```python
from build123d import *

# Parameters (mm, degrees)
BOSS_EXTRUDE1_DEPTH = 6.35
CUT_EXTRUDE1_DEPTH  = 6.35


with BuildPart() as part:
    # Sketch1 → Boss-Extrude1 (new body)
    with BuildSketch(Plane(origin=(0, 0, 0), x_dir=(1, 0, 0), z_dir=(0, 1, 0))):
        Polygon((14.834988784, -10.387570976), (18.04126264, 1.578405957), (12.8058292, 12.8058292), (1.578405957, 18.04126264), (-10.387570976, 14.834988784), (-17.493088004, 4.687258804), (-16.413394741, -7.653691664), (-7.653691664, -16.413394741), (4.687258804, -17.493088004), align=None)
    extrude(amount=BOSS_EXTRUDE1_DEPTH)

    # Sketch2 → Cut-Extrude1 (cut)
    with BuildSketch(Plane(origin=(0, 6.35, 0), x_dir=(1, 0, 0), z_dir=(0, 1, 0))):
        Polygon((1.833087105, 3.175), (-1.833087105, 3.175), (-3.666174209, 0), (-1.833087105, -3.175), (1.833087105, -3.175), (3.666174209, 0), align=None)
    extrude(amount=-CUT_EXTRUDE1_DEPTH, mode=Mode.SUBTRACT)


solid = part.part
```
The listing builds one solid part. Answer for the finished solid, in the listing's coordinates (mm). A direction names the side the tool comes from. Give positions to 0.01 mm unless a question says otherwise; leave off trailing zeros. Order: outer loops, then holes, each group sorted by start corner. A loop starts at its lowest first (then second) coordinate and runs counter-clockwise, first axis right, second up. Notation, with made-up numbers: (-21, 11.25) -> (30, 11.25) arc R12 cw to (30, 18.25) -> close; hole circle Ø7 at (79, -24). An arc over 180 degrees is marked (long way). Answer as a JSON object with one key per item and string values. Group by question number.
Item 1: Flat-ended cylindrical pins translate along their axes: pin 1 (1.5 mm diameter, centred on x = -7, y = 5.5, fed in from +Z); pin 2 (1.1 mm diameter, centred on x = -1, y = 3, fed in from +Z); pin 3 (2 mm diameter, centred on y = 5, z = -7.5, fed in from -X). Find the tip coordinate at first contact, or state that the pin passes through.
Item 2: The part is cut by section C-C on x = 6.5. Write down the section's boundary in (y, z), and give its area (3 significant figures).
Item 3: A tool of negligible diameter and unlimited length cuts with its end or side. For faces 5 (the flat face through (-2.76, 3.22, 1.57)), 6 (the flat face through (-13.89, 3.13, -9.83)), from which of +Z, -Z, +X, -X, +Y, -Y can it reach the whole face along a straight path? Write none if from no direction.
Item 4: The part is cut by section A-A on y = 0.5. Write down the section's boundary in (x, z) (3 decimals).
Item 5: The part is cut by section D-D on z = 11. Write down the section's boundary in (x, y).
Item 6: Consider L1, parallel to Z at x = -1, y = 2.5 (3 decimals); L2, parallel to Z at x = 2, y = 4; L3, parallel to X at y = 3.5, z = -10. Determine where each line is inside the solid, lowest interval first. Write a range as from..to.
Item 7: Determine the mould class of faces 1 (the flat face through (-16.96, 3.13, 1.4)), 2 (the flat face through (0, 3, -3.175)), 3 (the flat face through (15.46, 3.13, -7.11)), 4 (the flat face through (-4, 6.35, -1)) for opening direction Z: pulls with the +Z half, pulls with the -Z half, needs draft (parallel to the pull), parting line crosses it, or undercut.
Item 8: The part is cut by section B-B on x = -3. Write down the section's boundary in (y, z), and give its area (3 significant figures).
Result set:
{
 "1": {"pin 1": "z = 16.54", "pin 2": "z = 17.04", "pin 3": "x = -16.22"},
 "2": {"outline": "(0, -15.75) -> (6.35, -15.75) -> (6.35, 16.22) -> (0, 16.22) -> close", "area": "203 mm²"},
 "3": {"face 5": "+Y, -Y", "face 6": "-Z, -X, +Y, -Y"},
 "4": {"outline": "(-17.493, -4.687) -> (-10.388, -14.835) -> (1.578, -18.041) -> (12.806, -12.806) -> (18.041, -1.578) -> (14.835, 10.388) -> (4.687, 17.493) -> (-7.654, 16.413) -> (-16.413, 7.654) -> close; hole (-3.666, 0) -> (-1.833, -3.175) -> (1.833, -3.175) -> (3.666, 0) -> (1.833, 3.175) -> (-1.833, 3.175) -> close"},
 "5": {"outline": "(-13.07, 0) -> (13.96, 0) -> (13.96, 6.35) -> (-13.07, 6.35) -> close"},
 "6": {"L1": "-17.35..-3.175, 3.175..16.996", "L2": "-17.84..-2.89, 2.89..17.26", "L3": "-13.77..14.11"},
 "7": {"face 1": "pulls with the +Z half", "face 2": "undercut", "face 3": "pulls with the -Z half", "face 4": "needs draft"},
 "8": {"outline": "(0, -16.81) -> (6.35, -16.81) -> (6.35, -1.15) -> (0, -1.15) -> close; (0, 1.15) -> (6.35, 1.15) -> (6.35, 16.82) -> (0, 16.82) -> close", "area": "199 mm²"}
}
